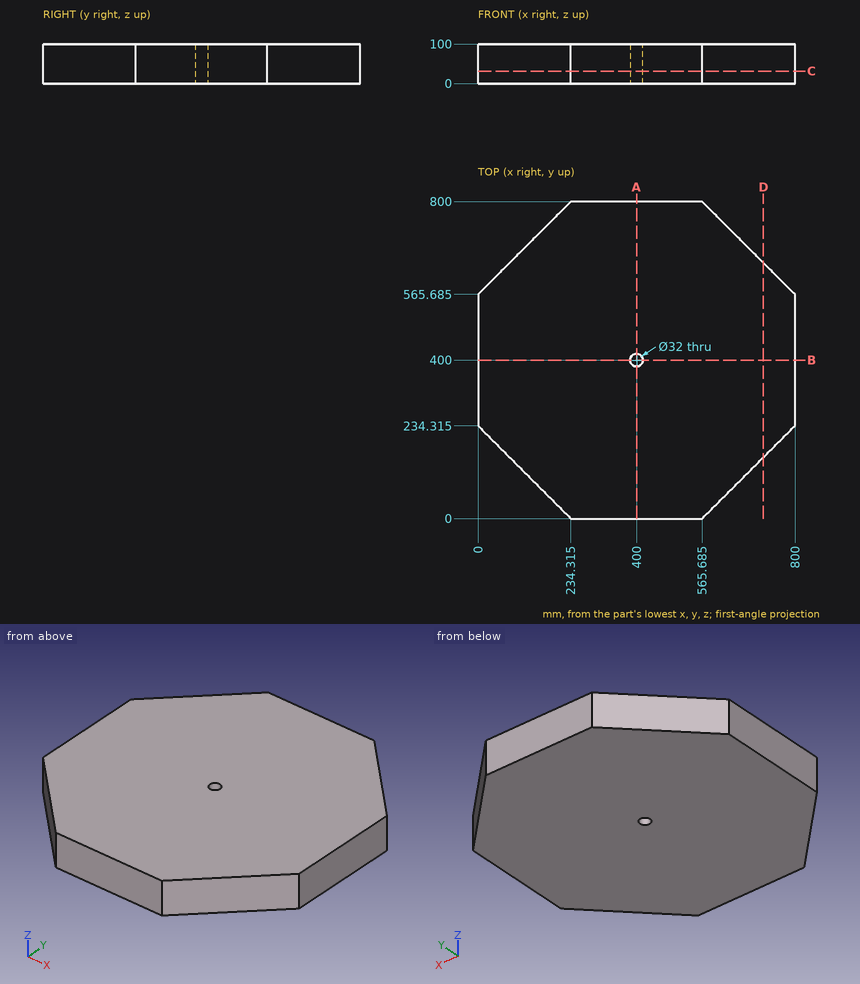
Geometry check sheet. Reference: drawing and pictorial views, mm from the part's lowest x, y, z. Coordinates: 2 decimals unless noted, no trailing zeros. Order: outer loops, then holes, each group sorted by start corner. A loop starts at its lowest first (then second) coordinate and runs counter-clockwise, first axis right, second up. Notation, with made-up numbers: (11, 77) - (33, 77) arc R22 cw to (33, 100) - close; hole circle Ø4 at (-5.75, 75.25). An arc over 180 degrees is marked (long way). Answer in a Markdown table with one row per item. Add a question column.
1) Cross-section at A-A, the plane x = 400. Record the cut outline in (y, z).
2) Cross-section at C-C, the plane z = 31.5. Record the cut outline in (x, y) (1 decimal).
3) Material ranges on line 1 along Y through (x, z) = (400, 51); line 2 along Y through (x, z) = (207, 7.5) (1 decimal), recorded low to high. Write a range as [from, to].
4) Cross-section at D-D, the plane x = 720. Record the cut outline in (y, z) (1 decimal), then the cut area to 3 significant figures.
5) Gauge pin test, flat ends, axial feed: P1, Ø1, axis at x = 135.5, z = 55, coming from the -Y side (1 decimal); P2, Ø5, axis at y = 589.5, z = 50, coming from the +X side (1 decimal); P3, Ø19, axis at x = 400, y = 400, coming from the +Z side. Record the tip position at first contact, or that the pin passes through.
Check result:
| question | item | result |
|---|---|---|
| 1 | outline | (0, 0) - (384, 0) - (384, 100) - (0, 100) - close; (416, 0) - (800, 0) - (800, 100) - (416, 100) - close |
| 2 | outline | (0, 234.3) - (234.3, 0) - (565.7, 0) - (800, 234.3) - (800, 565.7) - (565.7, 800) - (234.3, 800) - (0, 565.7) - close; hole circle Ø32 at (400, 400) |
| 3 | line 1 | y = [0, 384], [416, 800] |
| 3 | line 2 | y = [27.3, 772.7] |
| 4 | outline | (154.3, 0) - (645.7, 0) - (645.7, 100) - (154.3, 100) - close |
| 4 | area | 49,100 mm² |
| 5 | P1 | stops at y = 98.3 |
| 5 | P2 | stops at x = 778.7 |
| 5 | P3 | passes through |
